from build123d import *

# Parameters (mm, degrees)
SKETCH1_R           = 5.16
BOSS_EXTRUDE1_DEPTH = 1.5
SKETCH2_R           = 11
BOSS_EXTRUDE2_DEPTH = 3.5
SKETCH3_R           = 5.16
BOSS_EXTRUDE3_DEPTH = 16
SKETCH4_R           = 4
CUT_EXTRUDE1_DEPTH  = 26
SKETCH5_R           = 1.75
CUT_EXTRUDE2_DEPTH  = 26
CIRPATTERN1_COUNT   = 4
FILLET1_R           = 0.5
CHAMFER1_SIZE       = 0.5


with BuildPart() as part:
    # Sketch1 → Boss-Extrude1 (new body)
    with BuildSketch(Plane(origin=(0, 0, 0), x_dir=(1, 0, 0), z_dir=(0, 1, 0))):
        Circle(SKETCH1_R)
    extrude(amount=BOSS_EXTRUDE1_DEPTH)

    # Sketch2 → Boss-Extrude2 (add)
    with BuildSketch(Plane(origin=(0, 1.5, 0), x_dir=(1, 0, 0), z_dir=(0, 1, 0))):
        Circle(SKETCH2_R)
    extrude(amount=BOSS_EXTRUDE2_DEPTH)

    # Sketch3 → Boss-Extrude3 (add)
    with BuildSketch(Plane(origin=(0, 5, 0), x_dir=(1, 0, 0), z_dir=(0, 1, 0))):
        Circle(SKETCH3_R)
    extrude(amount=BOSS_EXTRUDE3_DEPTH)

    # Sketch4 → Cut-Extrude1 (cut)
    with BuildSketch(Plane(origin=(0, 21, 0), x_dir=(1, 0, 0), z_dir=(0, 1, 0))):
        Circle(SKETCH4_R)
    extrude(amount=-CUT_EXTRUDE1_DEPTH, mode=Mode.SUBTRACT)

    # Sketch5 → Cut-Extrude2 (cut)
    with BuildSketch(Plane(origin=(0, 5, 0), x_dir=(1, 0, 0), z_dir=(0, 1, 0))):
        with Locations((0, 8)):
            Circle(SKETCH5_R)
    cut_extrude2 = extrude(amount=-CUT_EXTRUDE2_DEPTH, mode=Mode.SUBTRACT)

    # CirPattern1: Cut-Extrude2 ×4 about axis
    cirpattern1_axis = Axis((0, 0, 0), (0, 1, 0))
    for i in range(1, CIRPATTERN1_COUNT):
        add(cut_extrude2.rotate(cirpattern1_axis, i * 360 / CIRPATTERN1_COUNT), mode=Mode.SUBTRACT)

    # Fillet1
    fillet1_edges = [part.edges().sort_by_distance(p)[0] for p in [
        (-5.16, 1.5, 0),
        (-11, 1.5, 0),
        (-11, 5, 0),
        (-5.16, 5, 0),
    ]]
    fillet(fillet1_edges, radius=FILLET1_R)

    # Chamfer1
    chamfer1_edges = [part.edges().sort_by_distance(p)[0] for p in [
        (-5.16, 21, 0),
        (-4, 0, 0),
        (-4, 21, 0),
        (-5.16, 0, 0),
    ]]
    chamfer(chamfer1_edges, length=CHAMFER1_SIZE)


solid = part.part
Design review of the part built by this model. Coordinates are the model's own, in mm. A direction names the side the tool comes from. Give positions to 0.01 mm unless a question says otherwise; leave off trailing zeros. Write each loop counter-clockwise with the first axis right and the second up, starting at its lowest first coordinate (ties: lowest second). Pieces come first, ordered by that corner, then holes. Notation, with made-up numbers: M 13.5,2.5 L 57.5,2.5 A21 ccw 57.5,14.5 Z; hole C -15.75,-6.5 d7. An arc over 180 degrees is marked long. Return JSON: item names as keys, results as strings. Group by question number.
Item 1: Take a section at B-B (z = 0). Count the separate pieces of the cut face and the enclosed holes in it, plus the area to 3 significant figures.
Item 2: Clearance check with flat-ended pins moving along their axes: pin 1 Ø5 at (x, y) = (-5.5, 10.5) entering from +Z; pin 2 Ø6 at (x, z) = (-5.5, -8.5) entering from +Y; pin 3 Ø1 at (x, z) = (2.5, -6) entering from -Y. State where each tip first meets the part, or that it passes through.
Item 3: The part is to be moulded in two halves that separate along Z. For faces 1 (the cylindrical face through (-0.867, 10.64, 3.905)), 2 (the cylindrical face through (-4.095, 0.746, 3.14)), 3 (the flat face through (5, 5, 5)), 4 (the cylindrical face through (0.228, 3.274, 9.735)), say which applies: pulls with the +Z half, pulls with the -Z half, needs draft (parallel to the pull), parting line crosses it, or undercut.
Item 4: Wall thickness on line 1 along X through (y, z) = (2.8, 0); line 2 along X through (y, z) = (13, 0.25): over which ranges is each line inside the solid? List them lowest first.
Item 5: Take a section at A-A (y = 3.25). Give the boundary of the cut face in (x, z), plus the area to 3 significant figures.
Item 6: Tool access review of faces 5 (the flat face through (5, 1.5, 5)), 6 (the cylindrical face through (-4.095, 12.895, 3.14)), 7 (the cylindrical face through (-2.38, 3.23, 10.74)): name each direction out of +Z, -Z, +X, -X, +Y, -Y from which nothing blocks a thin tool from reaching the whole face with its end or side.
Item 7: Take a section at D-D (y = 18.25). Give the boundary of the cut face in (x, z), plus the area to 3 significant figures.
Return value:
{
 "1": {"separate pieces": "4", "enclosed holes": "0", "area": "64.1 mm2"},
 "2": {"pin 1": "stops at z = 4.2", "pin 2": "stops at y = 5", "pin 3": "stops at y = 1.5"},
 "3": {"face 1": "undercut", "face 2": "parting line crosses it", "face 3": "needs draft", "face 4": "undercut"},
 "4": {"line 1": "x = -11 to -9.75, -6.25 to -4, 4 to 6.25, 9.75 to 11", "line 2": "x = -5.15 to -3.99, 3.99 to 5.15"},
 "5": {"outline": "C 0,0 d22; hole C -8,0 d3.5; hole C 0,0 d8; hole C 0,-8 d3.5; hole C 0,8 d3.5; hole C 8,0 d3.5", "area": "291 mm2"},
 "6": {"face 5": "-Y", "face 6": "+Y", "face 7": "+Y, -Y"},
 "7": {"outline": "C 0,0 d10.32; hole C 0,0 d8", "area": "33.4 mm2"}
}
